Source: CAD feature listing. Evaluate the final solid. Frame: model axes, mm. Coordinates: 2 decimals unless noted, no trailing zeros. Write each loop counter-clockwise with the first axis right and the second up, starting at its lowest first coordinate (ties: lowest second). Pieces come first, ordered by that corner, then holes. Notation, with made-up numbers: M -9.75,63 L 23.25,63 A16 cw 23.25,83 Z; hole C 80,-4 d5. An arc over 180 degrees is marked long. Answer as CSV lines item,"result". Start each with the question number.
1. Section C-C on y = 1.1. Count the separate pieces of the cut face and the enclosed holes in it, plus the area to 3 significant figures.
2. Line query: probe 1 along Z at (x, y) = (-14.5, 1.4); probe 2 along Z at (x, y) = (-1, 0.5); probe 3 along Z at (x, y) = (24, 1.2). Output: solid intervals per line, ascending. Write a range as [from, to].
3. Section A-A on z = 20. Return the cut outline in (x, y), plus the area to 3 significant figures.
4. Section B-B on x = -4. Return the cut outline in (y, z).
5. Contact query for flat-ended pins moving along their axis: pin 1 Ø6 at (x, z) = (61.95, 137.02) entering from +Y; pin 2 Ø0.5 at (y, z) = (1, 82.5) entering from -X; pin 3 Ø3.5 at (x, z) = (32.68, 7.09) entering from -Y. Output: stop coordinate, or through.
6. Section D-D on z = 88. Return the cut outline in (x, y), plus the area to 3 significant figures.
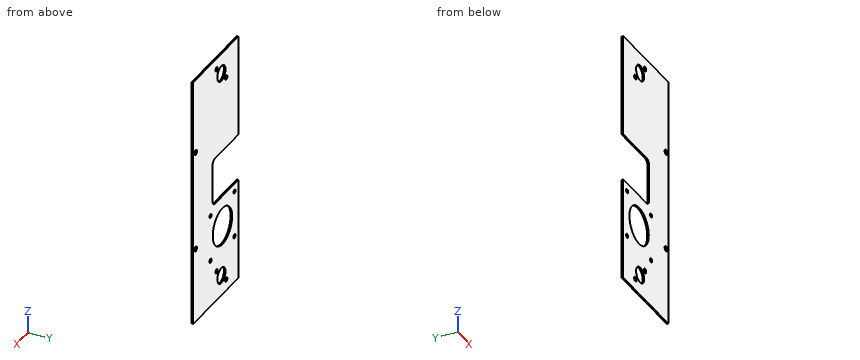
```python
from build123d import *

# Parameters (mm, degrees)
SKETCH1_R                 = 19.05
SKETCH1_R_2               = 7.9375
SKETCH1_R_3               = 2.062114731
BOSS_EXTRUDE1_DEPTH       = 1.5875
F_10_CLEARANCE_HOLE1_D    = 5.1054
F_8_CLEARANCE_HOLE1_D     = 4.4958
F_8_CLEARANCE_HOLE1_DEPTH = 6.35
F_8_CLEARANCE_HOLE1_TIP   = 1.350674586


with BuildPart() as part:
    # Sketch1 → Boss-Extrude1 (new body)
    with BuildSketch(Plane(origin=(0, 0, 0), x_dir=(1, 0, 0), z_dir=(0, 1, 0))):
        with BuildLine():
            Line((-22.186740071, -110.035971993), (-22.186740071, -213.413971993))
            Line((-22.186740071, -213.413971993), (66.713259929, -213.413971993))
            Line((66.713259929, -213.413971993), (66.713259929, 40.967028007))
            Line((66.713259929, 40.967028007), (-22.186740071, 40.967028007))
            Line((-22.186740071, 40.967028007), (-22.186740071, -62.410971993))
            Line((-22.186740071, -62.410971993), (23.850759929, -62.410971993))
            ThreePointArc((23.850759929, -62.410971993), (27.218355974, -63.805875948), (28.613259929, -67.173471993))
            Line((28.613259929, -67.173471993), (28.613259929, -105.273471993))
            ThreePointArc((28.613259929, -105.273471993), (27.218355974, -108.641068039), (23.850759929, -110.035971993))
            Line((23.850759929, -110.035971993), (-22.186740071, -110.035971993))
        make_face()
        with Locations(Location((9.106059929, -30.660971993, 0), (0, 0, 270))):
            Circle(SKETCH1_R, mode=Mode.SUBTRACT)
        with Locations(Location((11.150759929, 20.139028007, 0), (0, 0, 270))):
            Circle(SKETCH1_R_2, mode=Mode.SUBTRACT)
        with Locations(Location((11.150759929, -192.585971993, 0), (0, 0, 270))):
            Circle(SKETCH1_R_2, mode=Mode.SUBTRACT)
        with Locations(Location((-14.465140071, -7.089771993, 0), (0, 0, 270))):
            Circle(SKETCH1_R_3, mode=Mode.SUBTRACT)
        with Locations(Location((32.677259929, -7.089771993, 0), (0, 0, 90))):
            Circle(SKETCH1_R_3, mode=Mode.SUBTRACT)
        with Locations(Location((32.677259929, -54.232171993, 0), (0, 0, 270))):
            Circle(SKETCH1_R_3, mode=Mode.SUBTRACT)
        with Locations(Location((-14.465140071, -54.232171993, 0), (0, 0, 90))):
            Circle(SKETCH1_R_3, mode=Mode.SUBTRACT)
    extrude(amount=BOSS_EXTRUDE1_DEPTH)

    # #10 Clearance Hole1 (through all)
    with Locations(Plane(origin=(0, 1.5875, 0), x_dir=(1, 0, 0), z_dir=(0, 1, 0))):
        with Locations((61.950759929, -137.023471993), (61.950759929, -35.423471993)):
            Hole(F_10_CLEARANCE_HOLE1_D / 2)

    # #8 Clearance Hole1
    with Locations(Plane(origin=(0, 1.5875, 0), x_dir=(1, 0, 0), z_dir=(0, 1, 0))):
        with Locations((1.625759929, 29.664028007), (20.675759929, 10.614028007), (1.625759929, -183.060971993), (20.675759929, -202.110971993)):
            Hole(F_8_CLEARANCE_HOLE1_D / 2, depth=F_8_CLEARANCE_HOLE1_DEPTH)
            with Locations((0, 0, -(F_8_CLEARANCE_HOLE1_DEPTH + F_8_CLEARANCE_HOLE1_TIP / 2))):  # 118° drill point
                Cone(0, F_8_CLEARANCE_HOLE1_D / 2, F_8_CLEARANCE_HOLE1_TIP, mode=Mode.SUBTRACT)


solid = part.part
```
Values:
1,separate pieces,"1"
1,enclosed holes,"13"
1,area,"18,500 mm²"
2,probe 1,"[-40.97, 5.03], [9.15, 52.17], [56.29, 62.41], [110.04, 213.41]"
2,probe 2,"[-40.97, 14.51], [46.81, 62.41], [110.04, 213.41]"
2,probe 3,"[-40.97, 18.78], [42.54, 62.41], [110.03, 213.41]"
3,outline,"M -22.19,0 L -6.68,0 L -6.68,1.59 L -22.19,1.59 Z; M 24.89,0 L 66.71,0 L 66.71,1.59 L 24.89,1.59 Z"
3,area,"91.0 mm²"
4,outline,"M 0,-40.97 L 1.59,-40.97 L 1.59,16.84 L 0,16.84 Z; M 0,44.49 L 1.59,44.49 L 1.59,62.41 L 0,62.41 Z; M 0,110.04 L 1.59,110.04 L 1.59,213.41 L 0,213.41 Z"
5,pin 1,"y = 1.59"
5,pin 2,"x = 28.61"
5,pin 3,"through"
6,outline,"M 28.61,0 L 66.71,0 L 66.71,1.59 L 28.61,1.59 Z"
6,area,"60.5 mm²"
